from build123d import *

# Parameters (mm, degrees)
SKETCH1_R           = 16.7894
BOSS_EXTRUDE1_DEPTH = 50.8
SKETCH2_R           = 4.5085
BOSS_EXTRUDE2_DEPTH = 6.35
CUT_EXTRUDE1_START  = -2.159
SKETCH3_R           = 24.9555
SKETCH3_R_2         = 16.7894
CUT_EXTRUDE1_DEPTH  = 2.159


with BuildPart() as part:
    # Sketch1 → Boss-Extrude1 (new body)
    with BuildSketch(Plane(origin=(0, 0, 0), x_dir=(0, 0, -1), z_dir=(1, 0, 0))):
        Circle(SKETCH1_R)
        Polygon((-2.822954141, -4.8895), (2.822954141, -4.8895), (5.645908282, 0), (2.822954141, 4.8895), (-2.822954141, 4.8895), (-5.645908282, 0), align=None, mode=Mode.SUBTRACT)
    extrude(amount=BOSS_EXTRUDE1_DEPTH)

    # Sketch2 → Boss-Extrude2 (add)
    with BuildSketch(Plane.ZY):
        with BuildLine():
            ThreePointArc((-24.7777, 33.02), (-30.605886223, 30.605886223), (-33.02, 24.7777))
            ThreePointArc((-33.02, 24.7777), (-32.634975747, 18.719636617), (-31.48609891, 12.759061339))
            ThreePointArc((-31.48609891, 12.759061339), (-29.8577, 0), (-31.48609891, -12.759061339))
            ThreePointArc((-31.48609891, -12.759061339), (-32.634975747, -18.719636617), (-33.02, -24.7777))
            ThreePointArc((-33.02, -24.7777), (-30.605886223, -30.605886223), (-24.7777, -33.02))
            ThreePointArc((-24.7777, -33.02), (-18.719636617, -32.634975747), (-12.759061339, -31.48609891))
            ThreePointArc((-12.759061339, -31.48609891), (0, -29.8577), (12.759061339, -31.48609891))
            ThreePointArc((12.759061339, -31.48609891), (18.719636617, -32.634975747), (24.7777, -33.02))
            ThreePointArc((24.7777, -33.02), (30.605886223, -30.605886223), (33.02, -24.7777))
            ThreePointArc((33.02, -24.7777), (32.634975747, -18.719636617), (31.48609891, -12.759061339))
            ThreePointArc((31.48609891, -12.759061339), (29.8577, 0), (31.48609891, 12.759061339))
            ThreePointArc((31.48609891, 12.759061339), (32.634975747, 18.719636617), (33.02, 24.7777))
            ThreePointArc((33.02, 24.7777), (30.605886223, 30.605886223), (24.7777, 33.02))
            ThreePointArc((24.7777, 33.02), (18.719636617, 32.634975747), (12.759061339, 31.48609891))
            ThreePointArc((12.759061339, 31.48609891), (0, 29.8577), (-12.759061339, 31.48609891))
            ThreePointArc((-12.759061339, 31.48609891), (-18.719636617, 32.634975747), (-24.7777, 33.02))
        make_face()
        with Locations((24.7777, 24.7777)):
            Circle(SKETCH2_R, mode=Mode.SUBTRACT)
        with Locations((-24.7777, 24.7777)):
            Circle(SKETCH2_R, mode=Mode.SUBTRACT)
        with Locations((-24.7777, -24.7777)):
            Circle(SKETCH2_R, mode=Mode.SUBTRACT)
        with Locations((24.7777, -24.7777)):
            Circle(SKETCH2_R, mode=Mode.SUBTRACT)
        Polygon((2.822954141, 4.8895), (-2.822954141, 4.8895), (-5.645908282, 0), (-2.822954141, -4.8895), (2.822954141, -4.8895), (5.645908282, 0), align=None, mode=Mode.SUBTRACT)
    extrude(amount=BOSS_EXTRUDE2_DEPTH)

    # Sketch3 → Cut-Extrude1 (cut)
    with BuildSketch(Plane(origin=(0, 0, 0), x_dir=(0, 0, -1), z_dir=(1, 0, 0)).offset(CUT_EXTRUDE1_START)):
        Circle(SKETCH3_R)
        Circle(SKETCH3_R_2, mode=Mode.SUBTRACT)
    extrude(amount=CUT_EXTRUDE1_DEPTH, mode=Mode.SUBTRACT)


solid = part.part
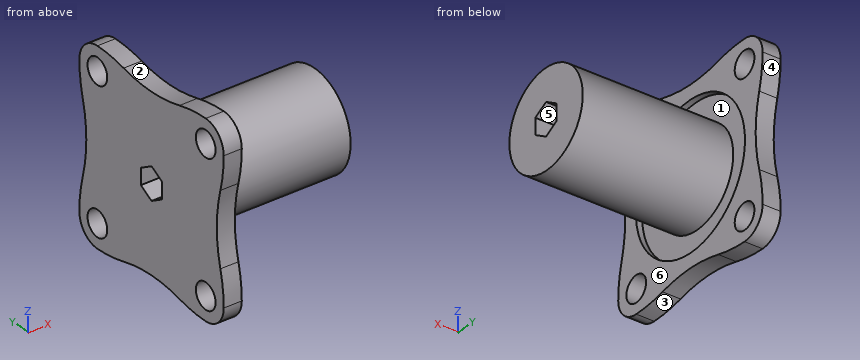
The model under review builds one solid part; all positions refer to its coordinate system, in mm. Face numbers are marked on the shaded views. A direction names the side the tool comes from. Give positions to 0.01 mm unless a question says otherwise; leave off trailing zeros. Order: outer loops, then holes, each group sorted by start corner. A loop starts at its lowest first (then second) coordinate and runs counter-clockwise, first axis right, second up. Notation, with made-up numbers: M -40,8.5 L 9,8.5 A14 cw 9,26.5 Z; hole C -29.5,81 d4. An arc over 180 degrees is marked long. Answer in a Markdown table with one row per item. Add a question column.
1. Add section B-B on x = 21.5. State the section outline as (y, z) points, plus the area to 3 significant figures.
2. To check wall thickness, follow line 1 along Y through (x, z) = (-0.8, 0); line 2 along Z through (x, y) = (-0.5, -23); line 3 along Z through (x, y) = (-2, 13). State the ranges of each line that lie inside material, in increasing order.
3. Add section A-A on z = 0. State the section outline as (x, y) points, plus the area to 3 significant figures.
4. Mouldability with a two-part tool opening along Z and no side actions: class the marked faces 1, 2 and 3 as released by +Z, released by -Z, zero draft, split by the parting line, or undercut.
5. Add section C-C on y = 18.5. State the section outline as (x, z) points.
6. Machinability: for the marked faces 4, 5 and 6, which of the approach directions +Z, -Z, +X, -X, +Y, -Y give a long, thin tool a straight path to every point of the face, cutting with its end or side? Answer none if there is none.
7. For pin 1 Ø11.5 at (y, z) = (24.78, -24.78) entering from -X; pin 2 Ø3 at (x, y) = (21, -4.5) entering from -Z; pin 3 Ø11.5 at (y, z) = (-24.78, -24.78) entering from +X; pin 4 Ø8 at (x, z) = (25, -3) entering from -Y, all flat-tipped, find the tip position at first contact; note any pin that passes through.
The answers:
| question | item | result |
|---|---|---|
| 1 | outline | C 0,0 d33.58; hole M -4.89,-2.82 L 0,-5.65 L 4.89,-2.82 L 4.89,2.82 L 0,5.65 L -4.89,2.82 Z |
| 1 | area | 803 mm2 |
| 2 | line 1 | -29.86 to -24.96, -16.79 to -4.89, 4.89 to 16.79, 24.96 to 29.86 |
| 2 | line 2 | -32.99 to -28.92, -20.63 to -9.68, 9.68 to 20.63, 28.92 to 32.99 |
| 2 | line 3 | -31.55 to -21.3, -10.62 to 10.62, 21.3 to 31.55 |
| 3 | outline | M -6.35,-29.86 L 0,-29.86 L 0,-24.96 L -2.16,-24.96 L -2.16,-16.79 L 50.8,-16.79 L 50.8,-4.89 L -6.35,-4.89 Z; M -6.35,4.89 L 50.8,4.89 L 50.8,16.79 L -2.16,16.79 L -2.16,24.96 L 0,24.96 L 0,29.86 L -6.35,29.86 Z |
| 3 | area | 1,490 mm2 |
| 4 | face 1 | undercut |
| 4 | face 2 | released by +Z |
| 4 | face 3 | released by -Z |
| 5 | outline | M -6.35,-32.61 L 0,-32.61 L 0,-16.75 L -2.16,-16.75 L -2.16,16.75 L 0,16.75 L 0,32.61 L -6.35,32.61 Z |
| 6 | face 4 | +X, -X, +Y |
| 6 | face 5 | +X, -X |
| 6 | face 6 | +X |
| 7 | pin 1 | x = -6.35 |
| 7 | pin 2 | z = -16.52 |
| 7 | pin 3 | x = 0 |
| 7 | pin 4 | y = -16.79 |
